The model under review builds one solid part; all positions refer to its coordinate system, in mm. Give positions to 0.01 mm unless a question says otherwise; leave off trailing zeros. Loops run counter-clockwise (first coordinate to the right, second up) from the corner with the lowest first, then second, coordinate; pieces in that order, holes last. Notation, with made-up numbers: (64, -3.75) - (88, -3.75) arc R10 cw to (88, 8.25) - close; hole circle Ø5 at (10.25, -17.75). An arc over 180 degrees is marked (long way). Answer as a JSON object with one key per item and string values.
from build123d import *

# Parameters (mm, degrees)
SKETCH_1_R      = 1
EXTRUDE_1_DEPTH = 1.5
FILLET_1_R      = 2


with BuildPart() as part:
    # 草图1 → 凸台-拉伸1 (new body)
    with BuildSketch(Plane(origin=(0, 0, 0), x_dir=(1, 0, 0), z_dir=(0, 1, 0))):
        with BuildLine():
            Line((-13.404756618, 11.25), (13.404756618, 11.25))
            ThreePointArc((13.404756618, 11.25), (15.151148095, 8.757437491), (16.439282223, 6))
            Line((16.439282223, 6), (16.439282223, -6))
            ThreePointArc((16.439282223, -6), (15.151148095, -8.757437491), (13.404756618, -11.25))
            Line((13.404756618, -11.25), (-13.404756618, -11.25))
            ThreePointArc((-13.404756618, -11.25), (-15.151148095, -8.757437491), (-16.439282223, -6))
            Line((-16.439282223, -6), (-16.439282223, 6))
            ThreePointArc((-16.439282223, 6), (-15.151148095, 8.757437491), (-13.404756618, 11.25))
        make_face()
        with Locations(Location((10.25, -8, 0), (0, 0, 270))):
            Circle(SKETCH_1_R, mode=Mode.SUBTRACT)
        with Locations(Location((-10.25, -8, 0), (0, 0, 90))):
            Circle(SKETCH_1_R, mode=Mode.SUBTRACT)
        with Locations(Location((-10.25, 8, 0), (0, 0, 270))):
            Circle(SKETCH_1_R, mode=Mode.SUBTRACT)
        with Locations(Location((10.25, 8, 0), (0, 0, 90))):
            Circle(SKETCH_1_R, mode=Mode.SUBTRACT)
    extrude(amount=EXTRUDE_1_DEPTH)

    # 圆角1
    fillet_1_edges = [part.edges().sort_by_distance(p)[0] for p in [
        (-13.404756618, 0.75, -11.25),
        (13.404756618, 0.75, -11.25),
        (16.439282223, 0.75, -6),
        (16.439282223, 0.75, 6),
        (13.404756618, 0.75, 11.25),
        (-13.404756618, 0.75, 11.25),
        (-16.439282223, 0.75, 6),
        (-16.439282223, 0.75, -6),
    ]]
    fillet(fillet_1_edges, radius=FILLET_1_R)


solid = part.part
Q1. The part is to be moulded in two halves that separate along X. For faces 1 (the face through (-13.324, 0.76, -11.043)), 2 (the face through (-9.26, 0.74, -8.13)), 3 (the face through (0, 0, 0)), 4 (the face through (11.24, 0.74, 7.87)), say which applies: +X half, -X half, draft (parallel to the pull), parting line (faces both ways), or undercut.
Results:
{"face 1": "-X half", "face 2": "undercut", "face 3": "draft", "face 4": "undercut"}
Q2. To check wall thickness, follow probe 1 along X at (y, z) = (0.3, -8); probe 2 along X at (y, z) = (1.3, 7.5); probe 3 along Z at (x, y) = (12.5, 1.3). State the ranges of each line that lie inside material, in increasing order. Write a range as [from, to].
Results:
{"probe 1": "x = [-15.56, -11.25], [-9.25, 9.25], [11.25, 15.56]", "probe 2": "x = [-15.81, -11.12], [-9.38, 9.38], [11.12, 15.81]", "probe 3": "z = [-11.25, 11.25]"}
Q3. Consider section D-D, the plane x = 13.5. State the section outline as (y, z) points, plus the area to 3 significant figures.
Results:
{"outline": "(0, -10.94) - (1.5, -10.94) - (1.5, 10.94) - (0, 10.94) - close", "area": "32.8 mm^2"}
Q4. Consider section C-C, the plane z = 8. State the section outline as (x, y) points.
Results:
{"outline": "(-15.56, 0) - (-11.25, 0) - (-11.25, 1.5) - (-15.56, 1.5) - close; (-9.25, 0) - (9.25, 0) - (9.25, 1.5) - (-9.25, 1.5) - close; (11.25, 0) - (15.56, 0) - (15.56, 1.5) - (11.25, 1.5) - close"}
Q5. Clearance check with a flat-ended pin moving along its axis: pin 1 Ø1.5 at (x, z) = (-10.5, 1.5) entering from -Y. State where the tip first meets the part, or that it passes through.
Results:
{"pin 1": "stops at y = 0"}
Q6. Consider section B-B, the plane y = 0.25. State the section outline as (x, z) points, plus the area to 3 significant figures.
Results:
{"outline": "(-16.44, -5.64) arc R2 ccw to (-16.3, -6.36) arc R17.5 ccw to (-14.04, -10.44) arc R2 ccw to (-12.44, -11.25) - (12.44, -11.25) arc R2 ccw to (14.04, -10.44) arc R17.5 ccw to (16.3, -6.36) arc R2 ccw to (16.44, -5.64) - (16.44, 5.64) arc R2 ccw to (16.3, 6.36) arc R17.5 ccw to (14.04, 10.44) arc R2 ccw to (12.44, 11.25) - (-12.44, 11.25) arc R2 ccw to (-14.04, 10.44) arc R17.5 ccw to (-16.3, 6.36) arc R2 ccw to (-16.44, 5.64) - close; hole circle Ø2 at (-10.25, -8); hole circle Ø2 at (-10.25, 8); hole circle Ø2 at (10.25, -8); hole circle Ø2 at (10.25, 8)", "area": "699 mm^2"}
Q7. Consider section A-A, the plane x = -10.25. State the section outline as (y, z) points, plus the area to 4 significant figures.
Results:
{"outline": "(0, -11.25) - (1.5, -11.25) - (1.5, -9) - (0, -9) - close; (0, -7) - (1.5, -7) - (1.5, 7) - (0, 7) - close; (0, 9) - (1.5, 9) - (1.5, 11.25) - (0, 11.25) - close", "area": "27.75 mm^2"}
